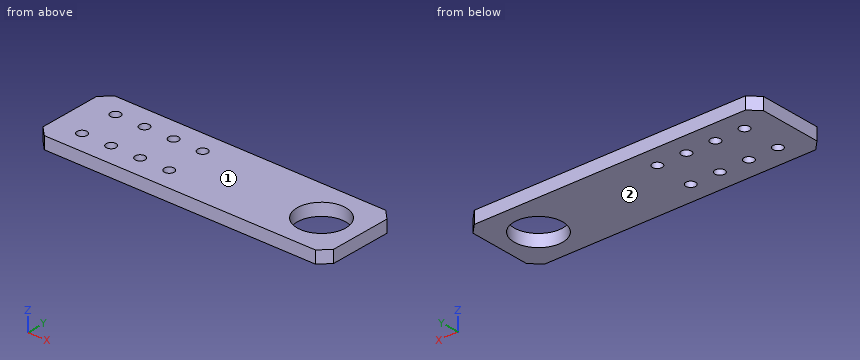
```python
from build123d import *

# Parameters (mm, degrees)
SKETCH1_W           = 200
SKETCH1_H           = 42
BOSS_EXTRUDE1_DEPTH = 6.35
SKETCH3_R           = 2
CUT_EXTRUDE2_DEPTH  = 103.378330227
SKETCH4_R           = 3.175
CUT_EXTRUDE3_DEPTH  = 103.378330227
CHAMFER1_SIZE       = 5
SKETCH9_R           = 3.175
CUT_EXTRUDE8_DEPTH  = 103.378330227
SKETCH10_R          = 12.5
CUT_EXTRUDE9_DEPTH  = 103.378330227
SKETCH12_R          = 3.302
CUT_EXTRUDE11_DEPTH = 103.378330227
SKETCH13_R          = 2
SKETCH13_R_2        = 3.302
SKETCH13_R_3        = 3.175
SKETCH13_R_4        = 2.54
CUT_EXTRUDE12_DEPTH = 10


with BuildPart() as part:
    # Sketch1 → Boss-Extrude1 (new body)
    with BuildSketch(Plane.XY):
        Rectangle(SKETCH1_W, SKETCH1_H)
    extrude(amount=BOSS_EXTRUDE1_DEPTH)

    # Sketch3 → Cut-Extrude2 (cut, through all)
    with BuildSketch(Plane.XY.offset(6.35)):
        with Locations((-55, 10)):
            Circle(SKETCH3_R)
        with Locations((-55, -10)):
            Circle(SKETCH3_R)
    extrude(amount=-CUT_EXTRUDE2_DEPTH, mode=Mode.SUBTRACT)

    # Sketch4 → Cut-Extrude3 (cut, through all)
    with BuildSketch(Plane.XY.offset(6.35)):
        with Locations((-76, 0)):
            Circle(SKETCH4_R)
    extrude(amount=-CUT_EXTRUDE3_DEPTH, mode=Mode.SUBTRACT)

    # Chamfer1
    chamfer1_edges = [part.edges().sort_by_distance(p)[0] for p in [
        (100, -21, 3.175),
        (-100, -21, 3.175),
        (-100, 21, 3.175),
        (100, 21, 3.175),
    ]]
    chamfer(chamfer1_edges, length=CHAMFER1_SIZE)

    # Sketch9 → Cut-Extrude8 (cut, through all)
    with BuildSketch(Plane.XY.offset(6.35)):
        with Locations((80, 0)):
            Circle(SKETCH9_R)
    extrude(amount=-CUT_EXTRUDE8_DEPTH, mode=Mode.SUBTRACT)

    # Sketch10 → Cut-Extrude9 (cut, through all)
    with BuildSketch(Plane.XY.offset(6.35)):
        with Locations((80, 0)):
            Circle(SKETCH10_R)
    extrude(amount=-CUT_EXTRUDE9_DEPTH, mode=Mode.SUBTRACT)

    # Sketch12 → Cut-Extrude11 (cut, through all)
    with BuildSketch(Plane.XY.offset(6.35)):
        with Locations((-93, 0)):
            Circle(SKETCH12_R)
    extrude(amount=-CUT_EXTRUDE11_DEPTH, mode=Mode.SUBTRACT)

    # Sketch13 → Cut-Extrude12 (cut)
    with BuildSketch(Plane.XY.offset(6.35)):
        Polygon((-50, -16), (-50, 16), (-45, 21), (-95, 21), (-100, 16), (-100, -16), (-95, -21), (-45, -21), align=None)
        with Locations((-55, -10)):
            Circle(SKETCH13_R, mode=Mode.SUBTRACT)
        with Locations((-93, 0)):
            Circle(SKETCH13_R_2, mode=Mode.SUBTRACT)
        with Locations((-76, 0)):
            Circle(SKETCH13_R_3, mode=Mode.SUBTRACT)
        with Locations((-55, 10)):
            Circle(SKETCH13_R, mode=Mode.SUBTRACT)
        with Locations((-35, 10)):
            Circle(SKETCH13_R_4)
        with Locations((-20, 10)):
            Circle(SKETCH13_R_4)
        with Locations((-5, 10)):
            Circle(SKETCH13_R_4)
        with Locations((10, 10)):
            Circle(SKETCH13_R_4)
        with Locations((-20, -10)):
            Circle(SKETCH13_R_4)
        with Locations((-5, -10)):
            Circle(SKETCH13_R_4)
        with Locations((10, -10)):
            Circle(SKETCH13_R_4)
        with Locations((-35, -10)):
            Circle(SKETCH13_R_4)
    extrude(amount=-CUT_EXTRUDE12_DEPTH, mode=Mode.SUBTRACT)


solid = part.part
```
For this review, take the finished solid that the model builds, in its own axes (mm). Face numbers are marked on the shaded views. Give positions to 0.01 mm unless a question says otherwise; leave off trailing zeros. Write each loop counter-clockwise with the first axis right and the second up, starting at its lowest first coordinate (ties: lowest second). Pieces come first, ordered by that corner, then holes. Notation, with made-up numbers: M 59,83.25 L 88,83.25 A29 cw 88,112.25 Z; hole C 3.5,-36.75 d1. An arc over 180 degrees is marked long. Answer as a JSON object with one key per item and string values. Group by question number.
Item 1: Consider section D-D on z = 4. Count the separate pieces of the cut face and the enclosed holes in it, plus the area to 3 significant figures.
Item 2: Consider section C-C on x = -35. Write out the cut boundary in (y, z).
Item 3: For probe 1 along Y at (x, z) = (10, 3.5); probe 2 along Y at (x, z) = (79.5, 5.25); probe 3 along Y at (x, z) = (73, 5.5), list the stretches that pass through material, from the lowest coordinate up. Write a range as [from, to].
Item 4: For pin 1 Ø3 at (x, y) = (-5, 10) entering from +Z; pin 2 Ø6.5 at (x, y) = (10, 10) entering from -Z, all flat-tipped, find the tip position at first contact; note any pin that passes through.
Item 5: Draft analysis for pull direction Z (two halves, no side actions). For the marked faces 1 and 2, state which applies: +Z half, -Z half, draft (parallel to the pull), parting line (faces both ways), or undercut.
Item 6: Consider section A-A on y = -10. Write out the cut boundary in (x, z).
Item 7: Consider section B-B on x = 80. Write out the cut boundary in (y, z), plus the area to 3 significant figures.
Check result:
{
 "1": {"separate pieces": "1", "enclosed holes": "9", "area": "5,600 mm^2"},
 "2": {"outline": "M -21,0 L -12.54,0 L -12.54,6.35 L -21,6.35 Z; M -7.46,0 L 7.46,0 L 7.46,6.35 L -7.46,6.35 Z; M 12.54,0 L 21,0 L 21,6.35 L 12.54,6.35 Z"},
 "3": {"probe 1": "y = [-21, -12.54], [-7.46, 7.46], [12.54, 21]", "probe 2": "y = [-21, -12.49], [12.49, 21]", "probe 3": "y = [-21, -10.36], [10.36, 21]"},
 "4": {"pin 1": "passes through", "pin 2": "stops at z = 0"},
 "5": {"face 1": "+Z half", "face 2": "-Z half"},
 "6": {"outline": "M -50,0 L -37.54,0 L -37.54,6.35 L -50,6.35 Z; M -32.46,0 L -22.54,0 L -22.54,6.35 L -32.46,6.35 Z; M -17.46,0 L -7.54,0 L -7.54,6.35 L -17.46,6.35 Z; M -2.46,0 L 7.46,0 L 7.46,6.35 L -2.46,6.35 Z; M 12.54,0 L 72.5,0 L 72.5,6.35 L 12.54,6.35 Z; M 87.5,0 L 100,0 L 100,6.35 L 87.5,6.35 Z"},
 "7": {"outline": "M -21,0 L -12.5,0 L -12.5,6.35 L -21,6.35 Z; M 12.5,0 L 21,0 L 21,6.35 L 12.5,6.35 Z", "area": "108 mm^2"}
}
